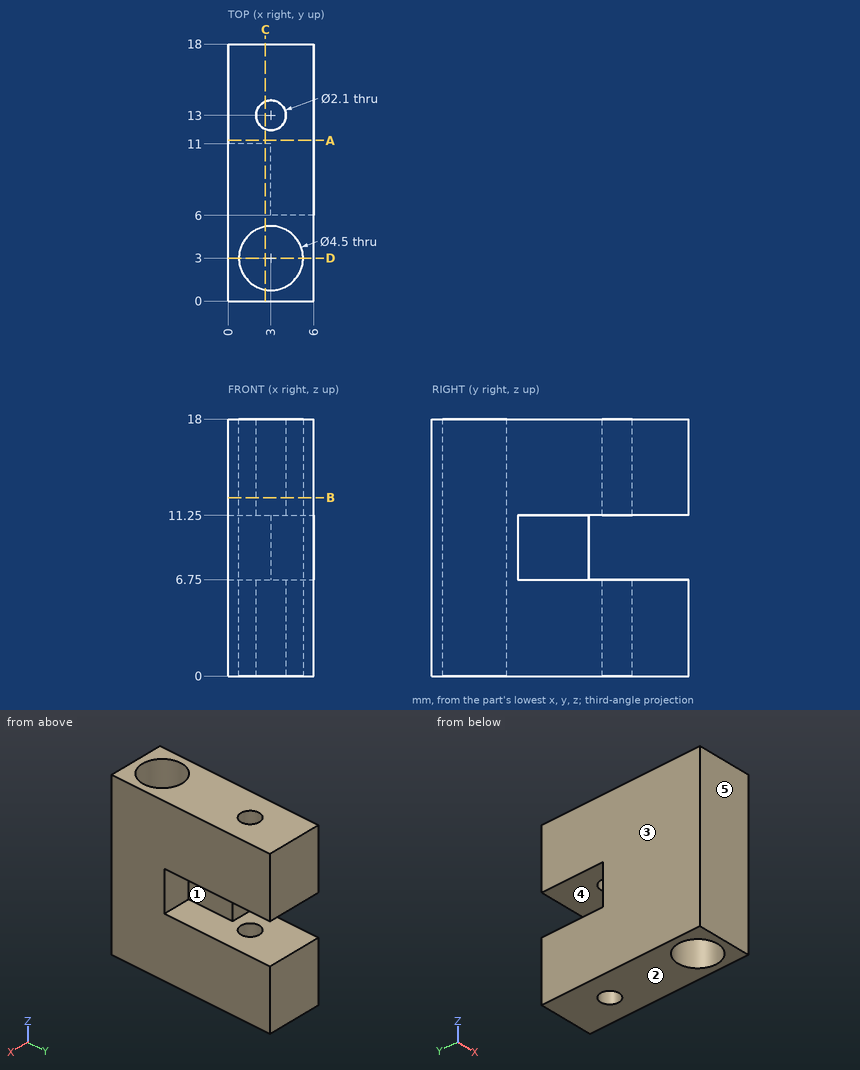
The drawing under review shows one solid part. Ordinate dimensions are in mm from its lowest x, y, z. A direction names the side the tool comes from. Coordinates: 2 decimals unless noted, no trailing zeros. Loops run counter-clockwise (first coordinate to the right, second up) from the corner with the lowest first, then second, coordinate; pieces in that order, holes last.
Item 1: Add section D-D (y = 3). Write out the cut boundary in (x, z), and give its area (3 significant figures).
Completed:
outline: (0, 0) - (0.75, 0) - (0.75, 18) - (0, 18) - close; (5.25, 0) - (6, 0) - (6, 18) - (5.25, 18) - close
area: 27.0 mm2
Item 2: Add section A-A (y = 11.25). Write out the cut boundary in (x, z).
Completed:
outline: (0, 0) - (6, 0) - (6, 6.75) - (0, 6.75) - close; (0, 11.25) - (6, 11.25) - (6, 18) - (0, 18) - close
Item 3: Wall thickness on L1, parallel to Y at x = 3, z = 15.75; L2, parallel to Z at x = 5.65, y = 13.25; L3, parallel to X at y = 13, z = 4.5: over which ranges is each line inside the solid? List them lowest first.
Completed:
L1: y = 0 to 0.75, 5.25 to 11.95, 14.05 to 18
L2: z = 0 to 6.75, 11.25 to 18
L3: x = 0 to 1.95, 4.05 to 6
Item 4: Add section C-C (x = 2.6). Write out the cut boundary in (y, z), and give its area (3 significant figures).
Completed:
outline: (0, 0) - (0.79, 0) - (0.79, 18) - (0, 18) - close; (5.21, 0) - (12.03, 0) - (12.03, 6.75) - (11, 6.75) - (11, 11.25) - (12.03, 11.25) - (12.03, 18) - (5.21, 18) - close; (13.97, 0) - (18, 0) - (18, 6.75) - (13.97, 6.75) - close; (13.97, 11.25) - (18, 11.25) - (18, 18) - (13.97, 18) - close
area: 187 mm2
Item 5: Draft analysis for pull direction Z (two halves, no side actions). For the marked faces 1, 2 and 3, state which applies: pulls with the +Z half, pulls with the -Z half, needs draft (parallel to the pull), parting line crosses it, or undercut.
Completed:
face 1: undercut
face 2: pulls with the -Z half
face 3: needs draft
Item 6: Clearance check with flat-ended pins moving along their axes: pin 1 (1.3 mm diameter, centred on y = 9, z = 8, fed in from +X); pin 2 (2.5 mm diameter, centred on x = 2, z = 9.5, fed in from +Y). State where each tip first meets the part, or that it passes through.
Completed:
pin 1: stops at x = 3
pin 2: stops at y = 11
Item 7: For the marked faces 4 and 5, list the 3-axis set-ups (+Z, -Z, +X, -X, +Y, -Y) from which the entire face can be reached by the end or side of a thin tool; tool diameter is ignored.
Completed:
face 4: +X, +Y
face 5: +Z, -Z, +X, -X, -Y
Item 8: Add section B-B (z = 12.5). Write out the cut boundary in (x, y), and give its area (3 significant figures).
Completed:
outline: (0, 0) - (6, 0) - (6, 18) - (0, 18) - close; hole circle Ø4.5 at (3, 3); hole circle Ø2.1 at (3, 13)
area: 88.6 mm2
